Verification items for the finished model (mm, model axes). Face numbers are marked on the shaded views. Coordinates: 2 decimals unless noted, no trailing zeros. Order: outer loops, then holes, each group sorted by start corner. A loop starts at its lowest first (then second) coordinate and runs counter-clockwise, first axis right, second up. Notation, with made-up numbers: M 81.25,82 L 105.25,82 A33 ccw 105.25,114 Z; hole C -36.75,63.5 d7. An arc over 180 degrees is marked long. Return JSON: item names as keys, results as strings.
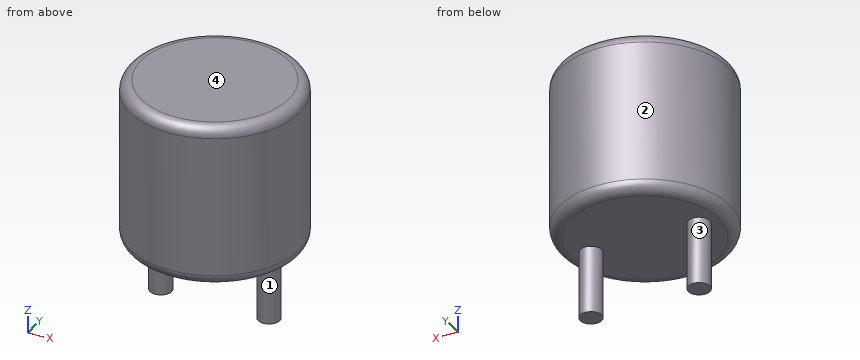
```python
from build123d import *

# Parameters (mm, degrees)
SKETCH001_R       = 0.5
PAD001_DEPTH      = 3.75
PAD001_DEPTH_BACK = 3.5
SKETCH_R          = 3.9
PAD_DEPTH         = 7.5
FILLET_R          = 0.5


with BuildPart() as pad001:
    # Sketch001 → Pad001 (new body, two sides)
    with BuildSketch(Plane.XY.offset(0.5)) as pad001_sk:
        Circle(SKETCH001_R)
        with Locations((5, 0)):
            Circle(SKETCH001_R)
    extrude(amount=PAD001_DEPTH)
    extrude(pad001_sk.sketch, amount=-PAD001_DEPTH_BACK)


with BuildPart() as obj1:
    # Sketch → Pad (new body)
    with BuildSketch(Plane.XY.offset(0.1)):
        with Locations((2.5, 0)):
            Circle(SKETCH_R)
    extrude(amount=PAD_DEPTH)

    # Fillet
    fillet_edges = [obj1.edges().sort_by_distance(p)[0] for p in [
        (-1.4, 0, 0.1),
        (-1.4, 0, 7.6),
    ]]
    fillet(fillet_edges, radius=FILLET_R)

    add(pad001.part)


solid = obj1.part
```
Q1. Draft check along X on the marked faces 1, 2, 3 and 4. Enter one of: pulls with the +X half, pulls with the -X half, needs draft (parallel to the pull), parting line crosses it, or undercut.
Values:
{"face 1": "undercut", "face 2": "parting line crosses it", "face 3": "undercut", "face 4": "needs draft"}
Q2. Go/stop test with flat-tipped pins: pin 1 (4 mm diameter, centred on y = 2.5, z = 2.5, fed in from +X); pin 2 (2 mm diameter, centred on y = 2.5, z = 1, fed in from +X); pin 3 (2 mm diameter, centred on x = 2, z = 2.5, fed in from -Y); pin 4 (1.5 mm diameter, centred on y = 1, z = 6, fed in from -X). Record where each tip stops, or that it passes through.
Values:
{"pin 1": "x = 6.37", "pin 2": "x = 6.1", "pin 3": "y = -3.9", "pin 4": "x = -1.39"}
Q3. Cross-section at C-C, the plane z = -0.75. Record the boundary of the cut face in (x, y).
Values:
{"outline": "C 0,0 d1; C 5,0 d1"}
Q4. Cross-section at B-B, the plane y = 0. Record the boundary of the cut face in (x, z), and give its area (3 significant figures).
Values:
{"outline": "M -1.4,0.6 A0.5 ccw -0.9,0.1 L -0.5,0.1 L -0.5,-3 L 0.5,-3 L 0.5,0.1 L 4.5,0.1 L 4.5,-3 L 5.5,-3 L 5.5,0.1 L 5.9,0.1 A0.5 ccw 6.4,0.6 L 6.4,7.1 A0.5 ccw 5.9,7.6 L -0.9,7.6 A0.5 ccw -1.4,7.1 Z", "area": "64.5 mm^2"}
Q5. Material ranges on line 1 along Z through (x, y) = (0.75, 0); line 2 along Y through (x, z) = (-0.5, 4.75); line 3 along Z through (x, y) = (4.5, 3.25), recorded low to high.
Values:
{"line 1": "0.1 to 7.6", "line 2": "-2.49 to 2.49", "line 3": "0.32 to 7.38"}
Q6. Cross-section at D-D, the plane z = 4. Record the boundary of the cut face in (x, y).
Values:
{"outline": "C 2.5,0 d7.8"}
Q7. Cross-section at A-A, the plane x = 2.5. Record the boundary of the cut face in (y, z), and give its area (3 significant figures).
Values:
{"outline": "M -3.9,0.6 A0.5 ccw -3.4,0.1 L 3.4,0.1 A0.5 ccw 3.9,0.6 L 3.9,7.1 A0.5 ccw 3.4,7.6 L -3.4,7.6 A0.5 ccw -3.9,7.1 Z", "area": "58.3 mm^2"}
